```python
from build123d import *

# Parameters (mm, degrees)
SKETCH2_OUTSIDE_W  = 11.446
SKETCH2_OUTSIDE_H  = 11.446
CUT_EXTRUDE1_DEPTH = 2


with BuildPart() as part:
    # Sketch1 → Revolve1 (revolve)
    with BuildSketch(Plane(origin=(0, 0, 0), x_dir=(0, 0, -1), z_dir=(1, 0, 0))):
        with BuildLine():
            Line((0, 7), (1.5, 7))
            Line((1.5, 7), (1.5, 0))
            Line((1.5, 0), (3, 0))
            Line((3, 0), (3, -1))
            Line((3, -1), (1, -1.352653961))
            Line((1, -1.352653961), (1, -3.208712153))
            ThreePointArc((1, -3.208712153), (2.447265782, -6.010774109), (0, -8))
            Line((0, -8), (0, 7))
        make_face()
    revolve(axis=Axis((0, -8, 0), (0, 1, 0)))

    # Sketch2 outside → Cut-Extrude1 (cut)
    with BuildSketch(Plane(origin=(0, 0, 0), x_dir=(1, 0, 0), z_dir=(0, 1, 0))):
        Rectangle(SKETCH2_OUTSIDE_W, SKETCH2_OUTSIDE_H)
        Polygon((1.443375673, 2.5), (-1.443375673, 2.5), (-2.886751346, 0), (-1.443375673, -2.5), (1.443375673, -2.5), (2.886751346, 0), align=None, mode=Mode.SUBTRACT)
    extrude(amount=-CUT_EXTRUDE1_DEPTH, mode=Mode.SUBTRACT)


solid = part.part
```
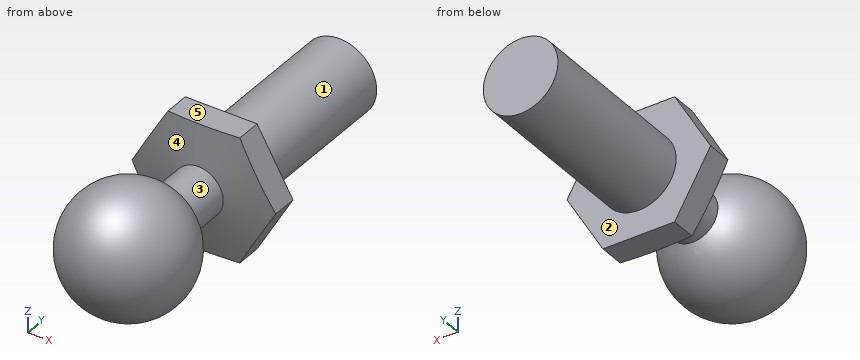
Read the model definition and answer for the solid it produces. Units are mm, in the model's axes. Face numbers are marked on the shaded views. A direction names the side the tool comes from. Give positions to 0.01 mm unless a question says otherwise; leave off trailing zeros. Order: outer loops, then holes, each group sorted by start corner. A loop starts at its lowest first (then second) coordinate and runs counter-clockwise, first axis right, second up.
(1) For a pull along Y with two mould halves and no side action, classify the marked faces 1, 2 and 3 as released by +Y, released by -Y, zero draft, split by the parting line, or undercut.
(2) Find section C-C (y = 5.75). Give the vertices of the cut face in (x, z).
(3) Given pin 1 (3 mm diameter, centred on y = 3.5, z = -1, fed in from +X), flat-ended and moving along its own axis, determine where the tip first touches the part or whether it passes through.
(4) Find section A-A (x = 0). Give the vertices of the cut face in (y, z), plus the area to 3 significant figures.
(5) For the marked faces 4 and 5, determine the directions among +Z, -Z, +X, -X, +Y, -Y from which every point of the face is accessible in a straight line to the end or side of a thin tool.
(6) Find section B-B (y = -2.75). Give the vertices of the cut face in (x, z), plus the area to 3 significant figures.
(7) Straight lines are drawn through the part: L1, parallel to Y at x = 0.4, z = -1.7; L2, parallel to Y at x = 0.6, z = -1.85; L3, parallel to X at y = 5.25, z = 0.05. For each, find the intervals that lie inside material, in ascending order.
Result sheet:
1. face 1: zero draft
1. face 2: released by +Y
1. face 3: undercut
2. outline: circle Ø3 at (0, 0)
3. pin 1: stops at x = 1.5
4. outline: (-3.21, -1) - (-1.35, -1) - (-1.09, -2.5) - (0, -2.5) - (0, -1.5) - (7, -1.5) - (7, 1.5) - (0, 1.5) - (0, 2.5) - (-1.09, 2.5) - (-1.35, 1) - (-3.21, 1) arc R2.5 ccw (long way) to start
4. area: 50.4 mm2
5. face 4: none
5. face 5: +Z, +X, -X, +Y, -Y
6. outline: circle Ø2 at (0, 0)
6. area: 3.14 mm2
7. L1: y = -7.29 to -3.71, -1.22 to 0
7. L2: y = -7.07 to -3.93, -1.19 to 0
7. L3: x = -1.5 to 1.5
